from build123d import *

# Parameters (mm, degrees)
SKETCH1_W             = 50.8
SKETCH1_H             = 76.2
BOSS_EXTRUDE1_DEPTH   = 100
SKETCH2_W             = 46.8
SKETCH2_H             = 72.2
CUT_EXTRUDE1_DEPTH    = 110.985317202
FILLET2_R             = 2
CORTAR_EXTRUIR2_DEPTH = 10
CROQUIS6_R            = 2.5
CORTAR_EXTRUIR6_DEPTH = 10
CROQUIS7_R            = 2.5
CORTAR_EXTRUIR7_DEPTH = 10
CROQUIS8_R            = 2.5
CORTAR_EXTRUIR8_DEPTH = 10


with BuildPart() as part:
    # Sketch1 → Boss-Extrude1 (new body)
    with BuildSketch(Plane(origin=(0, 0, 0), x_dir=(0, 0, -1), z_dir=(1, 0, 0))):
        Rectangle(SKETCH1_W, SKETCH1_H)
    extrude(amount=-BOSS_EXTRUDE1_DEPTH)

    # Sketch2 → Cut-Extrude1 (cut, through all)
    with BuildSketch(Plane(origin=(0, 0, 0), x_dir=(0, 0, -1), z_dir=(1, 0, 0))):
        Rectangle(SKETCH2_W, SKETCH2_H)
    extrude(amount=-CUT_EXTRUDE1_DEPTH, mode=Mode.SUBTRACT)

    # Fillet2
    fillet2_edges = [part.edges().sort_by_distance(p)[0] for p in [
        (-50, -36.1, 23.4),
        (-50, 36.1, 23.4),
        (-50, 36.1, -23.4),
        (-50, -36.1, -23.4),
        (-50, 38.1, 25.4),
        (-50, 38.1, -25.4),
        (-50, -38.1, -25.4),
        (-50, -38.1, 25.4),
    ]]
    fillet(fillet2_edges, radius=FILLET2_R)

    # Croquis2 → Cortar-Extruir2 (cut)
    with BuildSketch(Plane.XY.offset(25.4)):
        with BuildLine():
            ThreePointArc((-27, 26.5), (-30, 29.5), (-33, 26.5))
            Line((-33, 26.5), (-30, 26.5))
            Line((-30, 26.5), (-30, 23.5))
            ThreePointArc((-30, 23.5), (-27.878679656, 24.378679656), (-27, 26.5))
        make_face()
        with BuildLine():
            Line((-30, 26.5), (-33, 26.5))
            ThreePointArc((-33, 26.5), (-32.121320344, 24.378679656), (-30, 23.5))
            Line((-30, 23.5), (-30, 26.5))
        make_face()
        with BuildLine():
            ThreePointArc((-70, 23.5), (-67.878679656, 24.378679656), (-67, 26.5))
            Line((-67, 26.5), (-70, 26.5))
            Line((-70, 26.5), (-70, 23.5))
        make_face()
        with BuildLine():
            Line((-70, 26.5), (-67, 26.5))
            ThreePointArc((-67, 26.5), (-72.121320344, 28.621320344), (-70, 23.5))
            Line((-70, 23.5), (-70, 26.5))
        make_face()
        with BuildLine():
            ThreePointArc((-67, -26.5), (-67.878679656, -24.378679656), (-70, -23.5))
            Line((-70, -23.5), (-70, -26.5))
            Line((-70, -26.5), (-67, -26.5))
        make_face()
        with BuildLine():
            Line((-70, -26.5), (-70, -23.5))
            ThreePointArc((-70, -23.5), (-72.121320344, -28.621320344), (-67, -26.5))
            Line((-67, -26.5), (-70, -26.5))
        make_face()
        with BuildLine():
            ThreePointArc((-27, -26.5), (-27.878679656, -24.378679656), (-30, -23.5))
            Line((-30, -23.5), (-30, -26.5))
            Line((-30, -26.5), (-33, -26.5))
            ThreePointArc((-33, -26.5), (-30, -29.5), (-27, -26.5))
        make_face()
        with BuildLine():
            Line((-30, -26.5), (-30, -23.5))
            ThreePointArc((-30, -23.5), (-32.121320344, -24.378679656), (-33, -26.5))
            Line((-33, -26.5), (-30, -26.5))
        make_face()
    extrude(amount=-CORTAR_EXTRUIR2_DEPTH, mode=Mode.SUBTRACT)

    # Croquis6 → Cortar-Extruir6 (cut)
    with BuildSketch(Plane(origin=(0, 0, -25.4), x_dir=(-1, 0, 0), z_dir=(0, 0, -1))):
        with Locations(Location((17.2, 20, 0), (0, 0, 90))):
            Circle(CROQUIS6_R)
        with Locations(Location((17.2, -20, 0), (0, 0, 90))):
            Circle(CROQUIS6_R)
        with Locations(Location((41.2, -20, 0), (0, 0, 90))):
            Circle(CROQUIS6_R)
        with Locations(Location((41.2, 20, 0), (0, 0, 90))):
            Circle(CROQUIS6_R)
    extrude(amount=-CORTAR_EXTRUIR6_DEPTH, mode=Mode.SUBTRACT)

    # Croquis7 → Cortar-Extruir7 (cut)
    with BuildSketch(Plane.XZ.offset(38.1)):
        with Locations(Location((-15, 0.4, 0), (0, 0, 270))):
            Circle(CROQUIS7_R)
        with Locations(Location((-80, 0.4, 0), (0, 0, 270))):
            Circle(CROQUIS7_R)
    extrude(amount=-CORTAR_EXTRUIR7_DEPTH, mode=Mode.SUBTRACT)

    # Croquis8 → Cortar-Extruir8 (cut)
    with BuildSketch(Plane(origin=(0, 38.1, 0), x_dir=(1, 0, 0), z_dir=(0, 1, 0))):
        with Locations(Location((-90, 16, 0), (0, 0, 270))):
            Circle(CROQUIS8_R)
        with Locations(Location((-10, 16, 0), (0, 0, 270))):
            Circle(CROQUIS8_R)
        with Locations(Location((-90, -16, 0), (0, 0, 270))):
            Circle(CROQUIS8_R)
        with Locations(Location((-10, -16, 0), (0, 0, 270))):
            Circle(CROQUIS8_R)
    extrude(amount=-CORTAR_EXTRUIR8_DEPTH, mode=Mode.SUBTRACT)


solid = part.part
Geometry check sheet. Reference: the model listing, model coordinates, mm. A direction names the side the tool comes from. Coordinates: 2 decimals unless noted, no trailing zeros. Loops run counter-clockwise (first coordinate to the right, second up) from the corner with the lowest first, then second, coordinate; pieces in that order, holes last. Notation, with made-up numbers: (43, -31.75) - (80, -31.75) arc R11 ccw to (80, -21.75) - close; hole circle Ø8 at (80.5, 82). An arc over 180 degrees is marked (long way). Use one line per item in the form item = value. Start each with the question number.
Item 1: Gauge pin test, flat ends, axial feed: pin 1 (4 mm diameter, centred on x = -41.2, y = 20, fed in from -Z); pin 2 (3 mm diameter, centred on x = -90, z = -16, fed in from +Y). Record the tip position at first contact, or that the pin passes through.
Item 2: Thickness scan on probe 1 along X at (y, z) = (37.7, 16); probe 2 along X at (y, z) = (20, -24.25); probe 3 along Z at (x, y) = (-54.5, 15). Record the ranges inside material, lowest first.
Item 3: Mould release check, pull along Y, two halves, no side actions. Record for faces 5 (the face through (-77.52, -37.11, 0.73)), 6 (the face through (-18.7, 18, -24.4)), 7 (the face through (-49, -38.1, 0)): +Y half, -Y half, draft (parallel to the pull), parting line (faces both ways), or undercut.
Item 4: Section check B-B, the plane y = 20. Enter the section's corners in (x, z).
Item 5: Section check D-D, the plane z = 9. Enter the section's corners in (x, y).
Item 6: Section check A-A, the plane x = -90. Enter the section's corners in (y, z).
Item 7: Tool access check on faces 1 (the face through (-49, 0, 23.4)), 2 (the face through (-11.5, 37.1, 14)), 3 (the face through (-42.7, -22, -24.4)), 4 (the face through (-17.44, -37.11, 0.94)). Record the directions out of +Z, -Z, +X, -X, +Y, -Y that give a thin tool (end or side, any length) a straight path to the whole face; none if there is none.
Item 8: Section check C-C, the plane z = 0.4. Enter the section's corners in (x, y), and give its area (3 significant figures).
Computed:
q1.pin_1 = 23.4
q1.pin_2 = -36.1
q2.probe_1 = -100 to -92.5, -87.5 to -12.5, -7.5 to 0
q2.probe_2 = -100 to -43.7, -38.7 to -19.7, -14.7 to 0
q2.probe_3 = -25.4 to -23.4, 23.4 to 25.4
q3.face_5 = draft
q3.face_6 = undercut
q3.face_7 = -Y half
q4.outline = (-100, -25.4) - (-43.7, -25.4) - (-43.7, -23.4) - (-100, -23.4) - close; (-100, 23.4) - (0, 23.4) - (0, 25.4) - (-100, 25.4) - close; (-38.7, -25.4) - (-19.7, -25.4) - (-19.7, -23.4) - (-38.7, -23.4) - close; (-14.7, -25.4) - (0, -25.4) - (0, -23.4) - (-14.7, -23.4) - close
q5.outline = (-100, -38.1) - (0, -38.1) - (0, -36.1) - (-100, -36.1) - close; (-100, 36.1) - (0, 36.1) - (0, 38.1) - (-100, 38.1) - close
q6.outline = (-38.1, -23.4) arc R2 ccw to (-36.1, -25.4) - (36.1, -25.4) arc R2 ccw to (38.1, -23.4) - (38.1, -18.5) - (36.1, -18.5) - (36.1, -21.4) arc R2 cw to (34.1, -23.4) - (-34.1, -23.4) arc R2 cw to (-36.1, -21.4) - (-36.1, 21.4) arc R2 cw to (-34.1, 23.4) - (34.1, 23.4) arc R2 cw to (36.1, 21.4) - (36.1, 18.5) - (38.1, 18.5) - (38.1, 23.4) arc R2 ccw to (36.1, 25.4) - (-36.1, 25.4) arc R2 ccw to (-38.1, 23.4) - close; (36.1, -13.5) - (38.1, -13.5) - (38.1, 13.5) - (36.1, 13.5) - close
q7.face_1 = +X, -X
q7.face_2 = +Y
q7.face_3 = -Z
q7.face_4 = -Y
q8.outline = (-100, -38.1) - (-82.5, -38.1) - (-82.5, -36.1) - (-100, -36.1) - close; (-100, 36.1) - (0, 36.1) - (0, 38.1) - (-100, 38.1) - close; (-77.5, -38.1) - (-17.5, -38.1) - (-17.5, -36.1) - (-77.5, -36.1) - close; (-12.5, -38.1) - (0, -38.1) - (0, -36.1) - (-12.5, -36.1) - close
q8.area = 380 mm2
